Print and shaded views of the part. All mm, measured from the part's lowest x, y and z. Give positions to 0.01 mm unless a question says otherwise; leave off trailing zeros. Loops run counter-clockwise (first coordinate to the right, second up) from the corner with the lowest first, then second, coordinate; pieces in that order, holes last. Notation, with made-up numbers: (-39.75, -17.5) - (-24.75, -17.5) arc R25 cw to (-24.75, 21.5) - close; hole circle Ø9 at (-32, 62.25). An arc over 180 degrees is marked (long way). Return JSON: item names as keys, results as strings.
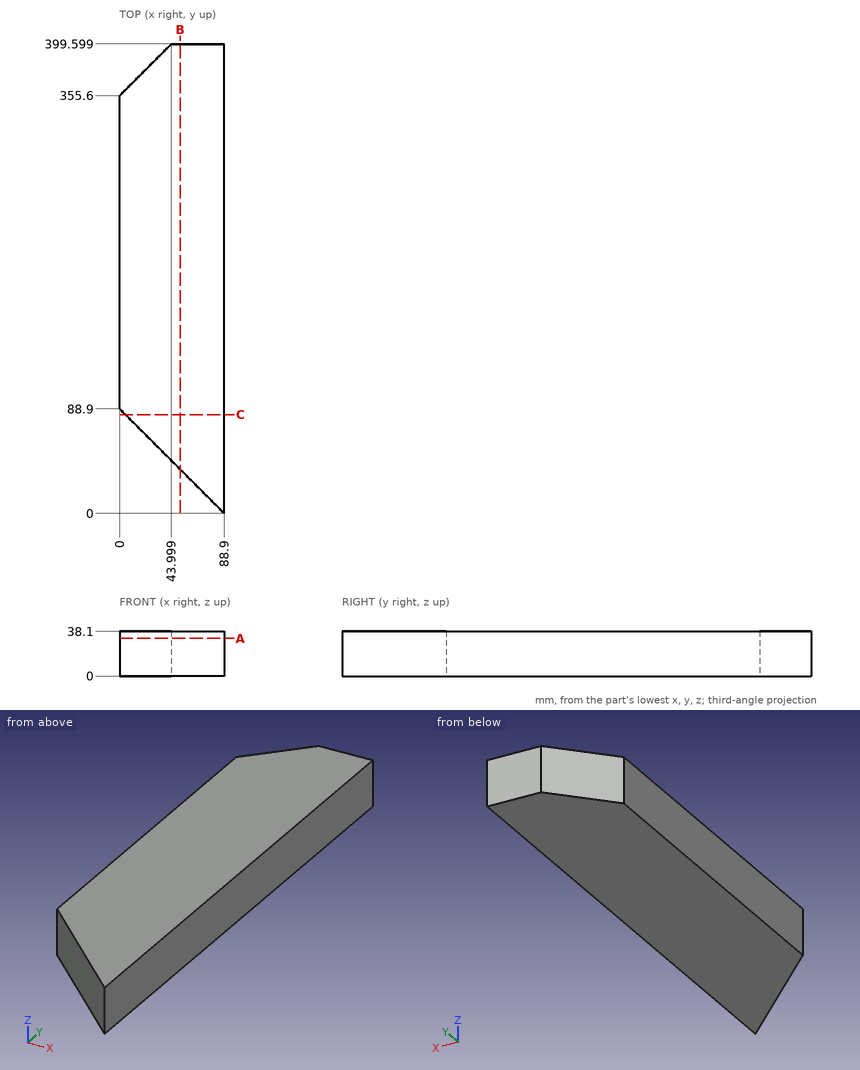
1. Drill centre lines: probe 1 along Y at (x, z) = (35.5, 10); probe 2 along X at (y, z) = (357, 32); probe 3 along Y at (x, z) = (6.5, 21.5). Where is each one in solid material? Low to high.
Values follow:
{"probe 1": "y = 53.4 to 391.1", "probe 2": "x = 1.4 to 88.9", "probe 3": "y = 82.4 to 362.1"}
2. Drop flat-ended pins along their axis: P1, Ø6, axis at x = 75.5, z = 6.5, coming from the -Y side; P2, Ø10, axis at x = 59, z = 4, coming from the -Y side. Give the stop position or say it passes through.
Values follow:
{"P1": "stops at y = 10.4", "P2": "stops at y = 24.9"}
3. Cut at C-C, the plane y = 84. Write the cut outline in (x, z), plus the area to 3 significant figures.
Values follow:
{"outline": "(4.9, 0) - (88.9, 0) - (88.9, 38.1) - (4.9, 38.1) - close", "area": "3,200 mm²"}
4. Cut at A-A, the plane z = 32. Write the cut outline in (x, y).
Values follow:
{"outline": "(0, 88.9) - (88.9, 0) - (88.9, 399.6) - (44, 399.6) - (0, 355.6) - close"}
5. Cut at B-B, the plane x = 51.5. Write the cut outline in (y, z), plus the area to 3 significant figures.
Values follow:
{"outline": "(37.4, 0) - (399.6, 0) - (399.6, 38.1) - (37.4, 38.1) - close", "area": "13,800 mm²"}
